```python
from build123d import *

# Parameters (mm, degrees)
BOSS_EXTRUDE1_DEPTH = 20
BOSS_EXTRUDE2_DEPTH = 25
SKETCH6_W           = 15
SKETCH6_H           = 15
BOSS_EXTRUDE3_DEPTH = 1.5


with BuildPart() as part:
    # Sketch2 → Boss-Extrude1 (new body)
    with BuildSketch(Plane(origin=(0, 0, 0), x_dir=(1, 0, 0), z_dir=(0, 1, 0))):
        Polygon((-35.179491924, -39.282032303), (-12.5, 0), (-12.5, 75), (0, 75), (0, 95), (-32.5, 95), (-32.5, 5.358983849), (-52.5, -29.282032303), align=None)
    boss_extrude1 = extrude(amount=BOSS_EXTRUDE1_DEPTH)

    # Mirror3: Boss-Extrude1 across plane
    add(boss_extrude1.mirror(Plane(origin=(0, 0, 0), x_dir=(0, 0, 1), z_dir=(1, 0, 0))))

    # Sketch4 → Boss-Extrude2 (add)
    with BuildSketch(Plane.ZY.offset(-12.5)):
        Polygon((-36.291651246, 0), (-27.631397208, 5), (-22.631397208, 5), (-13.97114317, 0), align=None)
    extrude(amount=BOSS_EXTRUDE2_DEPTH)

    # Sketch6 → Boss-Extrude3 (add)
    with BuildSketch(Plane.XZ):
        with Locations((-40, -55.645825623)):
            Rectangle(SKETCH6_W, SKETCH6_H)
        with Locations((40, -55.645825623)):
            Rectangle(SKETCH6_W, SKETCH6_H)
    extrude(amount=-BOSS_EXTRUDE3_DEPTH)


solid = part.part
```
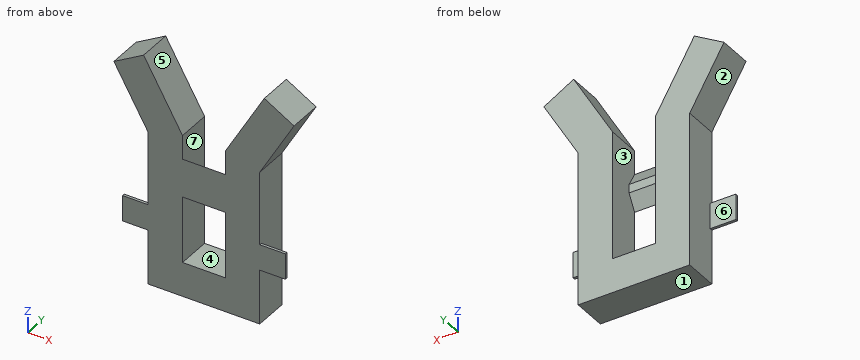
Work out the finished part from the listing and answer in its coordinate system (mm). Face numbers are marked on the shaded views. A direction names the side the tool comes from. Give positions to 0.01 mm unless a question says otherwise; leave off trailing zeros. Write each loop counter-clockwise with the first axis right and the second up, starting at its lowest first coordinate (ties: lowest second). Pieces come first, ordered by that corner, then holes.
(1) The part is cut by section A-A on z = -57.5. Write down the section's boundary in (x, y).
Final values:
outline: (-47.5, 0) - (-12.5, 0) - (-12.5, 20) - (-32.5, 20) - (-32.5, 1.5) - (-47.5, 1.5) - close; (12.5, 0) - (47.5, 0) - (47.5, 1.5) - (32.5, 1.5) - (32.5, 20) - (12.5, 20) - close
(2) The part is cut by section D-D on x = 42. Write down the section's boundary in (y, z).
Final values:
outline: (0, -63.15) - (1.5, -63.15) - (1.5, -48.15) - (0, -48.15) - close; (0, 11.1) - (20, 11.1) - (20, 35.34) - (0, 35.34) - close
(3) The part is cut by section C-C on y = 18.25. Write down the section's boundary in (x, z), plus the area to 3 significant figures.
Final values:
outline: (-52.5, 29.28) - (-32.5, -5.36) - (-32.5, -95) - (32.5, -95) - (32.5, -5.36) - (52.5, 29.28) - (35.18, 39.28) - (12.5, 0) - (12.5, -75) - (-12.5, -75) - (-12.5, 0) - (-35.18, 39.28) - close
area: 5,900 mm2
(4) The part is cut by section B-B on x = 4. Write down the section's boundary in (y, z).
Final values:
outline: (0, -95) - (20, -95) - (20, -75) - (0, -75) - close; (0, -36.29) - (5, -27.63) - (5, -22.63) - (0, -13.97) - close
(5) Flat-ended cylindrical pins translate along their axes: pin 1 Ø1.2 at (y, z) = (1, -56) entering from -X; pin 2 Ø1.2 at (x, y) = (-39.5, 1) entering from -Z; pin 3 Ø6 at (y, z) = (6.5, 21) entering from -X; pin 4 Ø1 at (x, z) = (33.5, 21) entering from -Y. Find the tip coordinate at first contact, or state that the pin passes through.
Final values:
pin 1: stops at x = -47.5
pin 2: stops at z = -63.15
pin 3: stops at x = -49.45
pin 4: stops at y = 0
(6) Straight lines are drawn through the part: line 1 (X direction, y = 10, z = -21.5); line 2 (Z direction, x = -5, y = 6.75); line 3 (X direction, y = 1.25, z = 12.5). For each, find the intervals that lie inside material, in ascending order.
Final values:
line 1: x = -32.5 to -12.5, 12.5 to 32.5
line 2: z = -95 to -75
line 3: x = -42.81 to -19.72, 19.72 to 42.81
(7) Which of the six approach directions +Z, -Z, +X, -X, +Y, -Y give full straight-line access (tool end or side, diameter ignored) to the marked faces 4, 5, 6 and 7?
Final values:
face 4: +Y, -Y
face 5: +Z, +Y, -Y
face 6: -Z, -X, +Y
face 7: +Y
(8) The mould has two halves that part along X. Classify the marked faces 1, 2 and 3: pulls with the +X half, pulls with the -X half, needs draft (parallel to the pull), parting line crosses it, or undercut.
Final values:
face 1: needs draft
face 2: pulls with the -X half
face 3: undercut
